Model file for the job. Use its own axes, mm. Face numbers are marked on the shaded views. A direction names the side the tool comes from. Give positions to 0.01 mm unless a question says otherwise; leave off trailing zeros. Loops run counter-clockwise (first coordinate to the right, second up) from the corner with the lowest first, then second, coordinate; pieces in that order, holes last. Notation, with made-up numbers: M 52.5,3 L 86.5,3 A15 cw 86.5,23 Z; hole C 20.5,6 d4. An arc over 180 degrees is marked long. Answer in a Markdown table with one row per item.
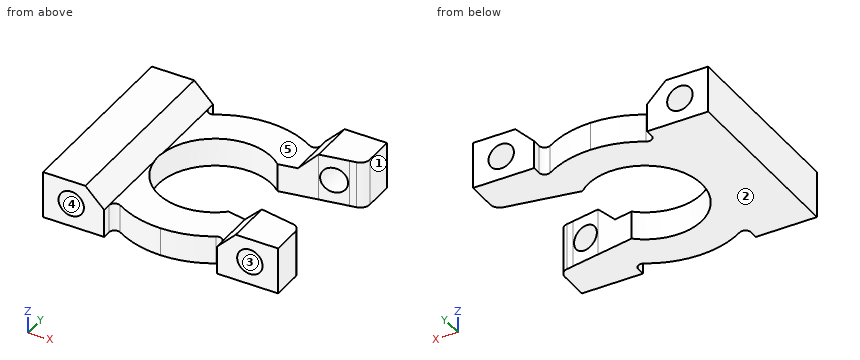
```python
from build123d import *

# Parameters (mm, degrees)
F0_W     = 1.5
F0_H     = 20
F0_W_2   = 3
F1_DEPTH = 5
F2_R     = 1.35
F3_DEPTH = 25
F5_DEPTH = 25
F6_R     = 0.6


with BuildPart() as f1:
    # F0 (on Top) → F1 (new body)
    with BuildSketch(Plane.XY):
        with BuildLine():
            ThreePointArc((4.0438224491, -4.5), (-6.05, 0), (4.0438224491, 4.5))
            Line((4.0438224491, 4.5), (8, 5.201766997))
            Line((8, 5.201766997), (8, 10))
            Line((8, 10), (-8, 10))
            Line((-8, 10), (-8, -10))
            Line((-8, -10), (8, -10))
            Line((8, -10), (8, -5.201766997))
            Line((8, -5.201766997), (4.0438224491, -4.5))
        make_face()
        Polygon((8, 10), (8, 5.201766997), (11, 5.7339223323), (11, 10), align=None)
        with BuildLine():
            Line((11, 10), (11, 5.7339223323))
            Line((11, 5.7339223323), (11.6746585367, 5.8535967123))
            ThreePointArc((11.6746585367, 5.8535967123), (12.2663741047, 6.1958312477), (12.5, 6.8382257772))
            Line((12.5, 6.8382257772), (12.5, 10))
            Line((12.5, 10), (11, 10))
        make_face()
        with BuildLine():
            Line((11.6746585367, -5.8535967123), (11, -5.7339223323))
            Line((11, -5.7339223323), (11, -10))
            Line((11, -10), (12.5, -10))
            Line((12.5, -10), (12.5, -6.8382257772))
            ThreePointArc((12.5, -6.8382257772), (12.2663741047, -6.1958312477), (11.6746585367, -5.8535967123))
        make_face()
        Polygon((11, -5.7339223323), (8, -5.201766997), (8, -10), (11, -10), align=None)
        with Locations((-11.75, 0)):
            Rectangle(F0_W, F0_H)
        with Locations((-9.5, 0)):
            Rectangle(F0_W_2, F0_H)
    extrude(amount=F1_DEPTH)

    # F2 (on face) → F3 (cut)
    with BuildSketch(Plane.XZ.offset(10)):
        with Locations((-9.5, 2.5)):
            Circle(F2_R)
        with Locations((9.5, 2.5)):
            Circle(F2_R)
        Polygon((8, 5), (0, 5), (-8, 5), (-6, 3), (0, 3), (6, 3), align=None)
    extrude(amount=-F3_DEPTH, mode=Mode.SUBTRACT)

    # F4 (on face) → F5 (cut)
    with BuildSketch(Plane.XY.offset(3)):
        with BuildLine():
            ThreePointArc((5.97e-08, 10), (3.1622776885, 9.4868329711), (6, 8))
            Line((6, 8), (6, 10))
            Line((6, 10), (5.97e-08, 10))
        make_face()
        with BuildLine():
            ThreePointArc((-6, 8), (-3.1622776319, 9.4868329899), (5.97e-08, 10))
            Line((5.97e-08, 10), (-6, 10))
            Line((-6, 10), (-6, 8))
        make_face()
        with BuildLine():
            Line((-6, -10), (5.97e-08, -10))
            ThreePointArc((5.97e-08, -10), (-3.1622776319, -9.4868329899), (-6, -8))
            Line((-6, -8), (-6, -10))
        make_face()
        with BuildLine():
            Line((5.97e-08, -10), (6, -10))
            Line((6, -10), (6, -8))
            ThreePointArc((6, -8), (3.1622776885, -9.4868329711), (5.97e-08, -10))
        make_face()
    extrude(amount=-F5_DEPTH, mode=Mode.SUBTRACT)

    # F6
    f6_edges = [f1.edges().sort_by_distance(p)[0] for p in [
        (-6, -8, 1.5),
        (-6, 8, 1.5),
        (6, 8, 1.5),
        (6, -8, 1.5),
    ]]
    fillet(f6_edges, radius=F6_R)


solid = f1.part
```
(1) Saw through at C-C, the plane z = 4.65. Give the cut face in (x, y), and give its area (3 significant figures).
Established:
| item | result |
|---|---|
| outline | M -12.5,-10 L -7.65,-10 L -7.65,10 L -12.5,10 Z; M 7.65,-10 L 12.5,-10 L 12.5,-6.84 A1 ccw 11.67,-5.85 L 7.65,-5.14 Z; M 7.65,5.14 L 11.67,5.85 A1 ccw 12.5,6.84 L 12.5,10 L 7.65,10 Z |
| area | 140 mm2 |
(2) Saw through at B-B, the plane x = -9.5. Give the cut face in (y, z), and give its area (3 significant figures).
Established:
| item | result |
|---|---|
| outline | M -10,0 L 10,0 L 10,1.15 L -10,1.15 Z; M -10,3.85 L 10,3.85 L 10,5 L -10,5 Z |
| area | 46.0 mm2 |
(3) Mould opens along Z. For the marked faces 1, 2 and 3 say: pulls with the +Z half, pulls with the -Z half, needs draft (parallel to the pull), parting line crosses it, or undercut.
Established:
| item | result |
|---|---|
| face 1 | needs draft |
| face 2 | pulls with the -Z half |
| face 3 | undercut |
(4) Which spindle directions (+Z, -Z, +X, -X, +Y, -Y) get a long thin tool onto all of the face, cutting with end or side? Do the marked faces 4 and 5. Say none if no direction does.
Established:
| item | result |
|---|---|
| face 4 | +Y, -Y |
| face 5 | +Z, +Y, -Y |
(5) Wall check: L1, parallel to Y at x = 0.25, z = 0.6; L2, parallel to X at y = -6.25, z = 3.65; L3, parallel to Z at x = 9.5, y = -8. Give the ranges that are in metal, low to high.
Established:
| item | result |
|---|---|
| L1 | y = -10 to -6.04, 6.04 to 10 |
| L2 | x = -12.5 to -10.21, -8.79 to -6.65, 6.65 to 8.79, 10.21 to 12.31 |
| L3 | z = 0 to 1.15, 3.85 to 5 |
(6) Saw through at A-A, the plane y = 0. Give the cut face in (x, z), and give its area (3 significant figures).
Established:
| item | result |
|---|---|
| outline | M -12.5,0 L -6.05,0 L -6.05,3.05 L -8,5 L -12.5,5 Z; hole C -9.5,2.5 d2.7 |
| area | 24.6 mm2 |
(7) Flat gauge pins, fed straight in: P1, Ø1, axis at x = 4.5, y = 2.5, coming from the -Z side; P2, Ø5, axis at x = -3.5, y = -5.5, coming from the -Z side; P3, Ø12, axis at x = -0.5, y = 8, coming from the +Z side; P4, Ø3, axis at y = -2.5, z = 3.5, coming from the +X side. Where does each tip first touch, or does it go through?
Established:
| item | result |
|---|---|
| P1 | passes through |
| P2 | stops at z = 0 |
| P3 | stops at z = 3.5 |
| P4 | stops at x = -4.61 |
(8) Saw through at D-D, the plane y = -7.25. Give the cut face in (x, z).
Established:
| item | result |
|---|---|
| outline | M -12.5,0 L 12.5,0 L 12.5,5 L 8,5 L 6,3 L -6,3 L -8,5 L -12.5,5 Z; hole C -9.5,2.5 d2.7; hole C 9.5,2.5 d2.7 |
